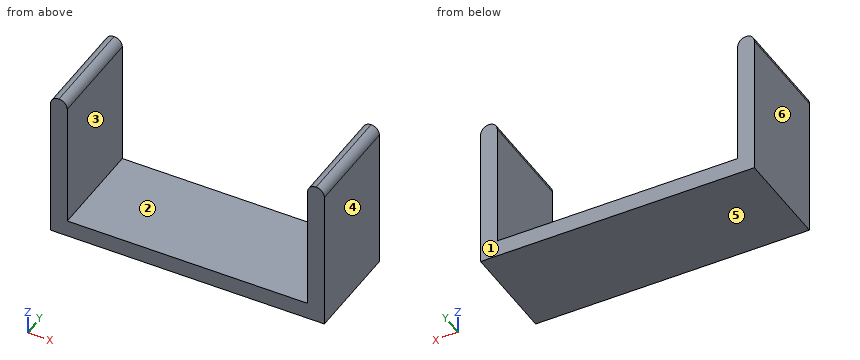
```python
from build123d import *

# Parameters (mm, degrees)
SKETCH_1_W      = 82
SKETCH_1_H      = 30
EXTRUDE_1_DEPTH = 5
SKETCH_2_W      = 5
SKETCH_2_H      = 30
EXTRUDE_2_DEPTH = 40
FILLET_1_R      = 2.5


with BuildPart() as part:
    # 草圖1 → 填料-伸長1 (new body)
    with BuildSketch(Plane.XY):
        with Locations((8.53492865, 4.8)):
            Rectangle(SKETCH_1_W, SKETCH_1_H)
    extrude(amount=EXTRUDE_1_DEPTH)

    # 草圖2 → 填料-伸長2 (add)
    with BuildSketch(Plane.XY.offset(5)):
        with Locations((-29.96507135, 4.8)):
            Rectangle(SKETCH_2_W, SKETCH_2_H)
        with Locations((47.03492865, 4.8)):
            Rectangle(SKETCH_2_W, SKETCH_2_H)
    extrude(amount=EXTRUDE_2_DEPTH)

    # 圓角1
    fillet_1_edges = [part.edges().sort_by_distance(p)[0] for p in [
        (44.53492865, 4.8, 45),
        (-27.46507135, 4.8, 45),
        (49.53492865, 4.8, 45),
        (-32.46507135, 4.8, 45),
    ]]
    fillet(fillet_1_edges, radius=FILLET_1_R - 0.0001)  # a hair under: the kernel refuses the full size


solid = part.part
```
Verification items for the finished model (mm, model axes). Face numbers are marked on the shaded views. A direction names the side the tool comes from. Give positions to 0.01 mm unless a question says otherwise; leave off trailing zeros. Order: outer loops, then holes, each group sorted by start corner. A loop starts at its lowest first (then second) coordinate and runs counter-clockwise, first axis right, second up. Notation, with made-up numbers: M 24,26 L 48,26 A7 cw 48,37 Z; hole C 35.5,57.5 d5. An arc over 180 degrees is marked long. Answer in a Markdown table with one row per item. Add a question column.
Item 1: Scan lines: probe 1 along X at (y, z) = (-2.75, 34.5); probe 2 along Z at (x, y) = (-17, 3.75). Record each from-to range of solid material in increasing order. Write a range as from..to.
Item 2: Section check A-A, the plane z = 22. Enter the section's corners in (x, y).
Item 3: Tool access check on the marked faces 1 and 2. Record the directions out of +Z, -Z, +X, -X, +Y, -Y that give a thin tool (end or side, any length) a straight path to the whole face; none if there is none.
Item 4: Gauge pin test, flat end, axial feed: pin 1 (1 mm diameter, centred on x = 24, y = 1, fed in from -Z). Record the tip position at first contact, or that the pin passes through.
Item 5: Section check C-C, the plane x = -5. Enter the section's corners in (y, z).
Item 6: Mould release check, pull along X, two halves, no side actions. Record for the marked faces 3, 4, 5 and 6: released by +X, released by -X, zero draft, split by the parting line, or undercut.
Filled sheet:
| question | item | result |
|---|---|---|
| 1 | probe 1 | x = -32.47..-27.47, 44.53..49.53 |
| 1 | probe 2 | z = 0..5 |
| 2 | outline | M -32.47,-10.2 L -27.47,-10.2 L -27.47,19.8 L -32.47,19.8 Z; M 44.53,-10.2 L 49.53,-10.2 L 49.53,19.8 L 44.53,19.8 Z |
| 3 | face 1 | +Z, -Z, +X, -X, +Y |
| 3 | face 2 | +Z, +Y, -Y |
| 4 | pin 1 | stops at z = 0 |
| 5 | outline | M -10.2,0 L 19.8,0 L 19.8,5 L -10.2,5 Z |
| 6 | face 3 | undercut |
| 6 | face 4 | released by +X |
| 6 | face 5 | zero draft |
| 6 | face 6 | released by -X |
